```python
from build123d import *

# Parameters (mm, degrees)
F1_DEPTH = 9
F3_DEPTH = 21
F4_R     = 7.5
F5_DEPTH = 37.3
F6_W     = 52.1081472671
F6_H     = 7
F7_DEPTH = 21
F9_DEPTH = 25


with BuildPart() as f1:
    # F0 (on Top) → F1 (new body)
    with BuildSketch(Plane.XY):
        with BuildLine():
            Line((61.1081472671, 0), (0, 0))
            ThreePointArc((0, 0), (-15, -15), (0, -30))
            Line((0, -30), (61.1081472671, -30))
            Line((61.1081472671, -30), (70.1081472671, -21))
            Line((70.1081472671, -21), (70.1081472671, -9))
            Line((70.1081472671, -9), (61.1081472671, 0))
        make_face()
    extrude(amount=F1_DEPTH)

    # F2 (on face) → F3 (join)
    with BuildSketch(Plane.XY.offset(9)):
        with BuildLine():
            Line((18, -30), (18, 0))
            Line((18, 0), (0, 0))
            ThreePointArc((0, 0), (-15, -15), (0, -30))
            Line((0, -30), (18, -30))
        make_face()
    extrude(amount=F3_DEPTH)

    # F4 (on face) → F5 (cut)
    with BuildSketch(Plane.XY.offset(30)):
        with Locations((0, -15)):
            Circle(F4_R)
    extrude(amount=-F5_DEPTH, mode=Mode.SUBTRACT)

    # F6 (on face) → F7 (join)
    with BuildSketch(Plane.XY.offset(9)):
        with Locations((44.0540736336, -15)):
            Rectangle(F6_W, F6_H)
    extrude(amount=F7_DEPTH)

    # F8 (on face) → F9 (cut)
    with BuildSketch(Plane.XZ.offset(18.5)):
        Polygon((70.1081472671, 30), (18, 30), (70.1081472671, 9), align=None)
    extrude(amount=-F9_DEPTH, mode=Mode.SUBTRACT)


solid = f1.part
```
Here's how the part is built. I have some questions about the finished solid (model axes, mm). A direction names the side the tool comes from. Coordinates: 2 decimals unless noted, no trailing zeros. Loops run counter-clockwise (first coordinate to the right, second up) from the corner with the lowest first, then second, coordinate; pieces in that order, holes last. Notation, with made-up numbers: (44, 77.25) - (81, 77.25) arc R27 cw to (81, 101.25) - close; hole circle Ø6 at (82.5, -22.5). An arc over 180 degrees is marked (long way). Return JSON: item names as keys, results as strings. Group by question number.
Item 1: If we section it at D-D on x = 50: Write out the boundary of the cut face in (y, z), and give its area (3 significant figures).
Item 2: Will these pins go through, and if not, where does the flat tip stop? P1, Ø12, axis at x = 45, z = 17, coming from the +Y side; P2, Ø6, axis at x = 48.5, y = -22.5, coming from the +Z side; P3, Ø10, axis at x = 60, y = -17, coming from the +Z side; P4, Ø1.5, axis at x = 52, z = 18, coming from the +Y side.
Item 3: I need wall thicknesses on line 1 (Y direction, x = 0, z = 21.25); line 2 (Y direction, x = 59, z = 12.5); line 3 (X direction, y = -16.75, z = 24.5). Which ranges of each line are inside material? Lowest first, please. Write a range as from..to.
Item 4: We'd pull the mould along X, two halves only. Please class faces 1 (the face through (-1.63, -22.32, 15.21)), 2 (the face through (18, -24, 19)), 3 (the face through (9, -15, 30)): +X half, -X half, draft (parallel to the pull), parting line (faces both ways), or undercut.
Item 5: If we section it at B-B on y = -15: Write out the boundary of the cut face in (x, z), and give its area (3 significant figures).
Item 6: On a 3-axis mill with a long thin cutter (end or side, diameter ignored), from which of +Z, -Z, +X, -X, +Y, -Y can I reach the whole of each face in a straight line? I mean faces 4 (the face through (27, -15, 0)), 5 (the face through (18, -6, 19)), 6 (the face through (38, -18.5, 17)). Say none if no direction works.
Item 7: If we section it at A-A on x = 4.5: Write out the boundary of the cut face in (y, z).
Item 8: If we section it at C-C on z = 25.75: Write out the boundary of the cut face in (x, y).
Calculated:
{
 "1": {"outline": "(-30, 0) - (0, 0) - (0, 9) - (-11.5, 9) - (-11.5, 17.1) - (-18.5, 17.1) - (-18.5, 9) - (-30, 9) - close", "area": "327 mm^2"},
 "2": {"P1": "stops at y = -11.5", "P2": "stops at z = 9", "P3": "stops at z = 15.09", "P4": "passes through"},
 "3": {"line 1": "y = -30..-22.5, -7.5..0", "line 2": "y = -18.5..-11.5", "line 3": "x = -14.9..-7.29, 7.29..31.65"},
 "4": {"face 1": "undercut", "face 2": "+X half", "face 3": "draft"},
 "5": {"outline": "(-15, 0) - (-7.5, 0) - (-7.5, 30) - (-15, 30) - close; (7.5, 0) - (70.11, 0) - (70.11, 9) - (18, 30) - (7.5, 30) - close", "area": "1,560 mm^2"},
 "6": {"face 4": "-Z, +X, -X, +Y, -Y", "face 5": "+Z, +X, +Y", "face 6": "+Z, +X, -Y"},
 "7": {"outline": "(-30, 0) - (-21, 0) - (-21, 30) - (-30, 30) - close; (-9, 0) - (0, 0) - (0, 30) - (-9, 30) - close"},
 "8": {"outline": "(0, -30) - (18, -30) - (18, -18.5) - (28.55, -18.5) - (28.55, -11.5) - (18, -11.5) - (18, 0) - (0, 0) arc R15 ccw to start; hole circle Ø15 at (0, -15)"}
}
